from build123d import *

# Parameters (mm, degrees)
ARRAY_COUNT   = 3
SKETCH_R      = 11
EXTRUDE_DEPTH = 4


with BuildPart() as array:
    # Sketch001 → Revolve (revolve)
    with BuildSketch(Plane.XZ):
        Polygon((0, 0), (0, 7), (5, 0), align=None)
    revolve(axis=Axis((0, 0, 4), (0, 0, 1)))

    # Array: Array ×3 about axis
    array_axis = Axis((-28, 0, 0), (0, 0, 1))


with BuildPart() as array_1:
    add(array.part)
    for i in range(1, ARRAY_COUNT):
        add(array.part.rotate(array_axis, i * 360 / ARRAY_COUNT))


with BuildPart() as array_2:
    # Array placement: moved
    add(array_1.part.moved(Location((28, 0, 4))))


with BuildPart() as fusion:
    # Sketch → Extrude (new body)
    with BuildSketch(Plane.XY):
        with BuildLine():
            Line((-19, 24.248711), (-19, -24.248711))
            ThreePointArc((-19, -24.248711), (-16.5, -28.578838), (-11.5, -28.578838))
            Line((-11.5, -28.578838), (30.5, -4.330127))
            ThreePointArc((30.5, -4.330127), (33, 0), (30.5, 4.330127))
            Line((30.5, 4.330127), (-11.5, 28.578838))
            ThreePointArc((-11.5, 28.578838), (-16.5, 28.578838), (-19, 24.248711))
        make_face()
        Circle(SKETCH_R, mode=Mode.SUBTRACT)
    extrude(amount=EXTRUDE_DEPTH)

    # Fusion: union Array
    add(array_2.part)


solid = fusion.part
Check sheet for the modelled part. Datum: model origin and axes. Units: mm. Coordinates: 2 decimals unless noted, no trailing zeros. Write each loop counter-clockwise with the first axis right and the second up, starting at its lowest first coordinate (ties: lowest second). Pieces come first, ordered by that corner, then holes.
Item 1: Cross-section at D-D on x = 16. Record the boundary of the cut face in (y, z), then the cut area to 3 significant figures.
Numbers:
outline: (-12.7, 0) - (12.7, 0) - (12.7, 4) - (-12.7, 4) - close
area: 102 mm2
Item 2: Mould release check, pull along X, two halves, no side actions. Record for faces 1 (the face through (26.58, 0.06, 9.01)), 2 (the face through (9.794, 16.285, 1.972)), 3 (the face through (0, -12, 4)), 4 (the face through (-2.38, -10.74, 1.97)): released by +X, released by -X, zero draft, split by the parting line, or undercut.
Numbers:
face 1: split by the parting line
face 2: released by +X
face 3: zero draft
face 4: undercut
Item 3: Depth check by flat-ended pin: pin 1 Ø1 at (x, z) = (-3.5, 1.5) entering from +Y; pin 2 Ø1.5 at (y, z) = (-23, 7.5) entering from +X; pin 3 Ø25 at (x, y) = (3.5, -9.5) entering from +Z. Enter the tip coordinate at first touch or a pass-through.
Numbers:
pin 1: stops at y = 24.25
pin 2: stops at x = -11.16
pin 3: stops at z = 4
Item 4: Cross-section at A-A on x = 0. Record the boundary of the cut face in (y, z).
Numbers:
outline: (-21.94, 0) - (-11, 0) - (-11, 4) - (-21.94, 4) - close; (11, 0) - (21.94, 0) - (21.94, 4) - (11, 4) - close
Item 5: Scan lines: probe 1 along Y at (x, z) = (0, 1.95); probe 2 along Y at (x, z) = (-8.5, 2.5); probe 3 along Z at (x, y) = (13, 10.5). Record each from-to range of solid material in increasing order.
Numbers:
probe 1: y = -21.94 to -11, 11 to 21.94
probe 2: y = -26.85 to -6.98, 6.98 to 26.85
probe 3: z = 0 to 4
Item 6: Cross-section at C-C on y = -18. Record the boundary of the cut face in (x, z).
Numbers:
outline: (-19, 0) - (6.82, 0) - (6.82, 4) - (-19, 4) - close
Item 7: Cross-section at B-B on z = 5.5. Record the boundary of the cut face in (x, y), then the cut area to 3 significant figures.
Numbers:
outline: circle Ø7.86 at (-14, -24.25); circle Ø7.86 at (-14, 24.25); circle Ø7.86 at (28, 0)
area: 145 mm2
